Design review of the part built by this model. Coordinates are the model's own, in mm. A direction names the side the tool comes from. Round coordinates to 2 decimals unless told otherwise and drop trailing zeros. Loops run counter-clockwise (first coordinate to the right, second up) from the corner with the lowest first, then second, coordinate; pieces in that order, holes last. Notation, with made-up numbers: (13.25, 87) - (19.25, 87) arc R21 cw to (19.25, 124) - close; hole circle Ø11 at (6, -10.75). An arc over 180 degrees is marked (long way). Use one line per item in the form item = value. Start each with the question number.
(1) We need section C-C, the plane z = 44. Write out the cut boundary in (x, y), then the cut area to 3 significant figures.
(2) For pin 1 (3 mm diameter, centred on x = 46.5, y = 3, fed in from +Z); pin 2 (12 mm diameter, centred on x = 145.5, y = 9, fed in from -Z); pin 3 (1 mm diameter, centred on x = 173.5, z = 82, fed in from +Y); pin 4 (3 mm diameter, centred on y = 5, z = 43.5, fed in from +X), all flat-tipped, find the tip position at first contact; note any pin that passes through.
(3) We need section D-D, the plane y = 8. Write out the cut boundary in (x, z), then the cut area to 3 significant figures.
(4) The part is to be moulded in two halves that separate along Z. For faces 1 (the cylindrical face through (107.89, -8.99, 147.03)), 2 (the cylindrical face through (237.065, -9.43, 117.085)), 3 (the flat face through (136, -10, 78)), 4 (the cylindrical face through (235.97, -7.399, 115.395)), say which applies: released by +Z, released by -Z, zero draft, split by the parting line, or undercut.
(5) Wall thickness on probe 1 along Z at (x, y) = (137.5, -5.3); probe 2 along Z at (x, y) = (9.5, -8.4); probe 3 along X at (y, z) = (-8.15, 52): over which ranges is each line inside the solid? List them lowest first. Write a range as [from, to].
(6) We need section B-B, the plane x = 137.5. Write out the cut boundary in (y, z), then the cut area to 3 significant figures.
(7) We need section A-A, the plane x = 67. Write out the cut boundary in (y, z), then the cut area to 3 significant figures.
(8) Machinability: for faces 5 (the cylindrical face through (134.64, -8.99, 10.4)), 6 (the flat face through (122, -4, 90)), which of the approach directions +Z, -Z, +X, -X, +Y, -Y give a long, thin tool a straight path to every point of the face, cutting with its end or side? Answer none if there is none.
from build123d import *

# Parameters (mm, degrees)
F1_DEPTH      = 10
F2_T          = -2
F5_DEPTH      = 4
F3_R          = 23.5
F6_DEPTH      = 8.001
F6_DEPTH_BACK = 2.001
F7_R          = 13.5
F8_DEPTH      = 20
F9_R          = 4
F10_DEPTH     = 20
F12_D         = 6
F13_R         = 2
F14_R         = 2


with BuildPart() as f1:
    # F0 (on Front) → F1 (new body)
    with BuildSketch(Plane.XZ):
        Polygon((0, 154), (0, 0), (275, 0), (275, 80), (201, 154), align=None)
    extrude(amount=F1_DEPTH)

    # F2
    f2_openings = [f1.faces().sort_by_distance(p)[0] for p in [
        (129.700907, 0, 73.382695),
    ]]
    offset(amount=F2_T, openings=f2_openings)

    # F4 (on face) → F5 (join)
    with BuildSketch(Plane(origin=(0, -8, 0), x_dir=(-1, 0, 0), z_dir=(0, 1, 0))):
        Polygon((-32, 87), (-32, 132), (-177, 132), (-177, 22), (-97, 22), align=None)
    extrude(amount=F5_DEPTH)

    # F3 (on face) → F6 (cut, two sides)
    with BuildSketch(Plane(origin=(0, -8, 0), x_dir=(-1, 0, 0), z_dir=(0, 1, 0))) as f6_sk:
        with Locations((-67, 102)):
            Circle(F3_R)
        with Locations((-137.5, 52)):
            Circle(F3_R)
    extrude(amount=F6_DEPTH, mode=Mode.SUBTRACT)
    extrude(f6_sk.sketch, amount=-F6_DEPTH_BACK, mode=Mode.SUBTRACT)

    # F7 (on face) → F8 (join)
    with BuildSketch(Plane(origin=(0, -8, 0), x_dir=(-1, 0, 0), z_dir=(0, 1, 0))):
        with Locations((-44, 44)):
            Circle(F7_R)
    extrude(amount=F8_DEPTH)

    # F9 (on face) → F10 (cut, through all)
    with BuildSketch(Plane(origin=(0, 12, 0), x_dir=(-1, 0, 0), z_dir=(0, 1, 0))):
        with Locations((-44, 44)):
            Circle(F9_R)
    extrude(amount=-F10_DEPTH, mode=Mode.SUBTRACT)

    # F12 (through all)
    with Locations(Plane.XZ.offset(10)):
        with Locations((9.5, 144.5), (109.5, 144.5), (231.2824855787, 110.2824855787), (265.5, 9.5), (137.5, 9.5), (9.5, 9.5)):
            Hole(F12_D / 2)

    # F13
    f13_edges = [f1.edges().sort_by_distance(p)[0] for p in [
        (0, -10, 77),
        (137.5, -10, 0),
        (238, -10, 117),
        (275, -10, 40),
        (275, -5, 0),
        (275, -5, 80),
        (201, -5, 154),
        (0, -5, 0),
        (100.5, -10, 154),
        (0, -5, 154),
    ]]
    fillet(f13_edges, radius=F13_R)

    # F14
    f14_edges = [f1.edges().sort_by_distance(p)[0] for p in [
        (273, -4, 2),
        (137.5, -8, 2),
        (273, -8, 40.585786),
        (236.585786, -8, 115.585786),
        (200.171573, -4, 152),
        (101.085786, -8, 152),
        (2, -4, 2),
        (2, -8, 77),
    ]]
    fillet(f14_edges, radius=F14_R)


solid = f1.part
Data:
q1.outline = (0, -8) arc R2 ccw to (2, -10) - (115.4, -10) - (115.4, -4) - (75, -4) - (75, -8) - (57.5, -8) - (57.5, 12) - (48, 12) - (48, -8) - (40, -8) - (40, 12) - (30.5, 12) - (30.5, -8) - (4, -8) arc R2 cw to (2, -6) - (2, 0) - (0, 0) - close; (159.6, -10) - (273, -10) arc R2 ccw to (275, -8) - (275, 0) - (273, 0) - (273, -6) arc R2 cw to (271, -8) - (177, -8) - (177, -4) - (159.6, -4) - close
q1.area = 1,100 mm^2
q2.pin_1 = 57.46
q2.pin_2 = through
q2.pin_3 = -4
q2.pin_4 = 57.5
q3.outline = circle Ø27 at (44, 44); hole circle Ø8 at (44, 44)
q3.area = 522 mm^2
q4.face_1 = undercut
q4.face_2 = released by +Z
q4.face_3 = zero draft
q4.face_4 = undercut
q5.probe_1 = [0, 2], [22, 28.5], [75.5, 132], [152, 154]
q5.probe_2 = [0.04, 6.5], [12.5, 141.5], [147.5, 153.96]
q5.probe_3 = [0.01, 114], [161, 274.99]
q6.outline = (-10, 2) arc R2 ccw to (-8, 0) - (0, 0) - (0, 2) - (-6, 2) arc R2 cw to (-8, 4) - (-8, 6.5) - (-10, 6.5) - close; (-10, 12.5) - (-8, 12.5) - (-8, 22) - (-4, 22) - (-4, 28.5) - (-10, 28.5) - close; (-10, 75.5) - (-4, 75.5) - (-4, 132) - (-8, 132) - (-8, 150) arc R2 cw to (-6, 152) - (0, 152) - (0, 154) - (-8, 154) arc R2 ccw to (-10, 152) - close
q6.area = 486 mm^2
q7.outline = (-10, 2) arc R2 ccw to (-8, 0) - (0, 0) - (0, 2) - (-6, 2) arc R2 cw to (-8, 4) - (-8, 52) - (-4, 52) - (-4, 78.5) - (-10, 78.5) - close; (-10, 125.5) - (-4, 125.5) - (-4, 132) - (-8, 132) - (-8, 150) arc R2 cw to (-6, 152) - (0, 152) - (0, 154) - (-8, 154) arc R2 ccw to (-10, 152) - close
q7.area = 378 mm^2
q8.face_5 = +Y, -Y
q8.face_6 = +Y
